Geometry: final body of the model. Coordinates: model frame, mm. A direction names the side the tool comes from. Round coordinates to 2 decimals unless told otherwise and drop trailing zeros. Loops run counter-clockwise (first coordinate to the right, second up) from the corner with the lowest first, then second, coordinate; pieces in that order, holes last. Notation, with made-up numbers: (-2.5, 0.5) - (52.5, 0.5) arc R34 cw to (52.5, 35.5) - close; hole circle Ø11 at (41.25, 69.5). An arc over 180 degrees is marked (long way). Answer as a JSON object with one key per item and string values. Group by question number.
Item 1: Reachability of faces 1 (the face through (-21, 3, 3.4)), 2 (the face through (18.314, 5.221, 1.676)) from +Z, -Z, +X, -X, +Y, -Y: full face, straight path, thin tool, end or side. Return the list, or none.
Item 2: Section A-A (z = 12). Return the cut outline in (x, y), plus the area to 3 significant figures.
Item 3: Section C-C (y = 5). Return the cut outline in (x, z).
Item 4: First-contact query: pin 1 (5 mm diameter, centred on x = -28.5, z = 13, fed in from +Y); pin 2 (3 mm diameter, centred on x = -1, y = 8, fed in from +Z); pin 3 (3 mm diameter, centred on x = 0.5, z = 12.5, fed in from -Y); pin 4 (3 mm diameter, centred on x = 20, y = 5, fed in from -Z). Flat tips, straight axial feed; report the tip coordinate or a pass-through.
Item 5: Line query: line 1 (X direction, y = 18, z = 8.9); line 2 (X direction, y = 18, z = 4.25); line 3 (Y direction, x = 20, z = 1.15). Output: solid intervals per line, ascending.
Item 6: Section D-D (x = 33). Return the cut outline in (y, z).
Item 7: Draft query along Y for faces 3 (the face through (0, 25, 16)), 4 (the face through (-23.47, 5.46, 3.89)), 5 (the face through (0, 25.5, 11)). Return one class per face: released by +Y, released by -Y, zero draft, split by the parting line, or undercut.
Item 8: Section B-B (x = -3.5). Return the cut outline in (y, z).
Autodesk Inventor part; units mm, degrees
ref_plane "YZ Plane" through (0, 0, 0) normal (1, 0, 0) x (0, 1, 0)
ref_plane "XZ Plane" through (0, 0, 0) normal (0, 1, 0) x (-1, 0, 0)
ref_plane "XY Plane" through (0, 0, 0) normal (0, 0, 1) x (1, 0, 0)
sketch "Skizze1" plane through (0, 0, 0) normal (0, 0, 1) x (1, 0, 0)
  line L0 (-20, 36) -> (20, 36)
  line L1 (38, 18) -> (38, 18)
  line L2 (20, 0) -> (-20, 0)
  line L3 (-38, 18) -> (-38, 18)
  arc A0 (-20, 36) -> (-38, 18) centre (-20, 18) ccw
  arc A1 (-38, 18) -> (-20, 0) centre (-20, 18) ccw
  arc A2 (38, 18) -> (20, 36) centre (20, 18) ccw
  arc A3 (20, 0) -> (38, 18) centre (20, 18) ccw
  point P0 (0, 0)
  point P1 (0, 0)
  point P2 (38, 18)
  dimension "d0" = 36
  dimension "d1" = 18
  dimension "d2" = 40
extrude "Extrusion1" add sketch "Skizze1" along normal blind 4.4
sketch "Skizze2" plane through (0, 0, 4.4) normal (0, 0, 1) x (1, 0, 0)
  line L0 (-11.25, 18) -> (11.25, 18) construction
  line L1 (-11.25, 23) -> (11.25, 23)
  line L2 (11.25, 13) -> (-11.25, 13)
  arc A0 (-11.25, 23) -> (-11.25, 13) centre (-11.25, 18) ccw
  arc A1 (11.25, 13) -> (11.25, 23) centre (11.25, 18) ccw
  arc A2 (-20, 36) -> (-20, 0) centre (-20, 18) ccw
  line L3 (-20, 0) -> (20, 0)
  line L4 (-20, 18) -> (20, 18) construction
  line L5 (-20, 10.5) -> (20, 10.5)
  line L6 (20, 25.5) -> (-20, 25.5)
  arc A3 (-20, 25.5) -> (-20, 10.5) centre (-20, 18) ccw
  arc A4 (20, 10.5) -> (20, 25.5) centre (20, 18) ccw
  point P0 (0, 0)
  point P1 (0, 18)
  point P2 (-38, 18)
  point P3 (0, 0)
  point P4 (0, 18)
  dimension "d5" = 22.5
  dimension "d6" = 5
  dimension "d7" = 7.5
extrude "Extrusion3" add sketch "Skizze2" along normal blind 5.6 contours L1 A1 L2 A0
extrude "Extrusion4" add sketch "Skizze2" along normal blind 11.6
fillet "Rundung1" radius 2 4 edges at (27.5, 18, 4.4) (0, 10.5, 4.4) (-27.5, 18, 4.4) (0, 25.5, 4.4)
sketch "Skizze3" plane through (0, 0, 10) normal (0, 0, 1) x (1, 0, 0)
  arc A0 (-11.25, 23) -> (-11.25, 13) centre (-11.25, 18) ccw
  point P0 (0, 0)
hole "Bohrung1" at (-11.25, 18, 10) direction (0, 0, -1) diameter 5 depth 10 counterbore diameter 7 counterbore depth 2
sketch "Skizze4" plane through (0, 0, 10) normal (0, 0, 1) x (1, 0, 0)
  arc A0 (11.25, 13) -> (11.25, 23) centre (11.25, 18) ccw
  point P0 (0, 0)
hole "Bohrung2" at (11.25, 18, 10) direction (0, 0, -1) diameter 5 depth 10 counterbore diameter 7 counterbore depth 2
sketch "Skizze5" plane through (0, 0, 4.4) normal (0, 0, 1) x (1, 0, 0)
  arc A0 (-20, 31) -> (-20, 5) centre (-20, 18) ccw construction
  line L0 (-20, 31) -> (20, 31) construction
  arc A1 (20, 10.5) -> (20, 25.5) centre (20, 18) ccw construction
  line L1 (20, 25.5) -> (-20, 25.5) construction
  arc A2 (-20, 25.5) -> (-20, 10.5) centre (-20, 18) ccw construction
  line L2 (-20, 10.5) -> (20, 10.5) construction
  line L3 (11.25, 13) -> (-11.25, 13) construction
  arc A3 (-11.25, 23) -> (-11.25, 13) centre (-11.25, 18) ccw construction
  line L4 (-11.25, 23) -> (11.25, 23) construction
  arc A4 (11.25, 13) -> (11.25, 23) centre (11.25, 18) ccw construction
  arc A5 (20, 5) -> (20, 31) centre (20, 18) ccw construction
  line L5 (-20, 5) -> (20, 5) construction
  arc A6 (-20, 27.5) -> (-20, 8.5) centre (-20, 18) ccw construction
  point P0 (0, 0)
  point P1 (20, 8.5)
  point P2 (-33, 18)
  point P3 (33, 18)
  dimension "d30" = 13
hole "Bohrung3" at (-33, 18, 4.4) at (33, 18, 4.4) at (-20, 31, 4.4) at (-20, 5, 4.4) at (20, 31, 4.4) at (20, 5, 4.4) direction (0, 0, -1) diameter 3.4 end through all counterbore diameter 7 counterbore depth 1
properties material "Stahl, galvanisiert"
Values:
{
 "1": {"face 1": "+Z", "face 2": "+Z, -Z"},
 "2": {"outline": "(-20, 10.5) - (20, 10.5) arc R7.5 ccw to (20, 25.5) - (-20, 25.5) arc R7.5 ccw to start; hole (-11.25, 13) - (11.25, 13) arc R5 ccw to (11.25, 23) - (-11.25, 23) arc R5 ccw to start", "area": "473 mm^2"},
 "3": {"outline": "(-32.45, 0) - (-21.7, 0) - (-21.7, 3.4) - (-23.5, 3.4) - (-23.5, 4.4) - (-32.45, 4.4) - close; (-18.3, 0) - (18.3, 0) - (18.3, 3.4) - (16.5, 3.4) - (16.5, 4.4) - (-16.5, 4.4) - (-16.5, 3.4) - (-18.3, 3.4) - close; (21.7, 0) - (32.45, 0) - (32.45, 4.4) - (23.5, 4.4) - (23.5, 3.4) - (21.7, 3.4) - close"},
 "4": {"pin 1": "stops at y = 22.5", "pin 2": "stops at z = 4.67", "pin 3": "stops at y = 10.5", "pin 4": "passes through"},
 "5": {"line 1": "x = -27.5 to -14.75, -7.75 to 7.75, 14.75 to 27.5", "line 2": "x = -38 to -36.5, -29.5 to -13.75, -8.75 to 8.75, 13.75 to 29.5, 36.5 to 38", "line 3": "y = 0 to 3.3, 6.7 to 29.3, 32.7 to 36"},
 "6": {"outline": "(5.55, 0) - (16.3, 0) - (16.3, 3.4) - (14.5, 3.4) - (14.5, 4.4) - (5.55, 4.4) - close; (19.7, 0) - (30.45, 0) - (30.45, 4.4) - (21.5, 4.4) - (21.5, 3.4) - (19.7, 3.4) - close"},
 "7": {"face 3": "zero draft", "face 4": "undercut", "face 5": "released by +Y"},
 "8": {"outline": "(0, 0) - (36, 0) - (36, 4.4) - (27.5, 4.4) arc R2 cw to (25.5, 6.4) - (25.5, 16) - (23, 16) - (23, 10) - (13, 10) - (13, 16) - (10.5, 16) - (10.5, 6.4) arc R2 cw to (8.5, 4.4) - (0, 4.4) - close"}
}
